Answer from the drawing. Dimensions are ordinates in mm from the lowest x, y and z of the part. A direction names the side the tool comes from. Coordinates: 2 decimals unless noted, no trailing zeros. Order: outer loops, then holes, each group sorted by start corner. A loop starts at its lowest first (then second) coordinate and runs counter-clockwise, first axis right, second up. Notation, with made-up numbers: (-23, 12) -> (14, 12) arc R30 ccw to (14, 39) -> close; hole circle Ø11 at (40.25, 52.25). An arc over 180 degrees is marked (long way). Answer in a Markdown table with one row per item.
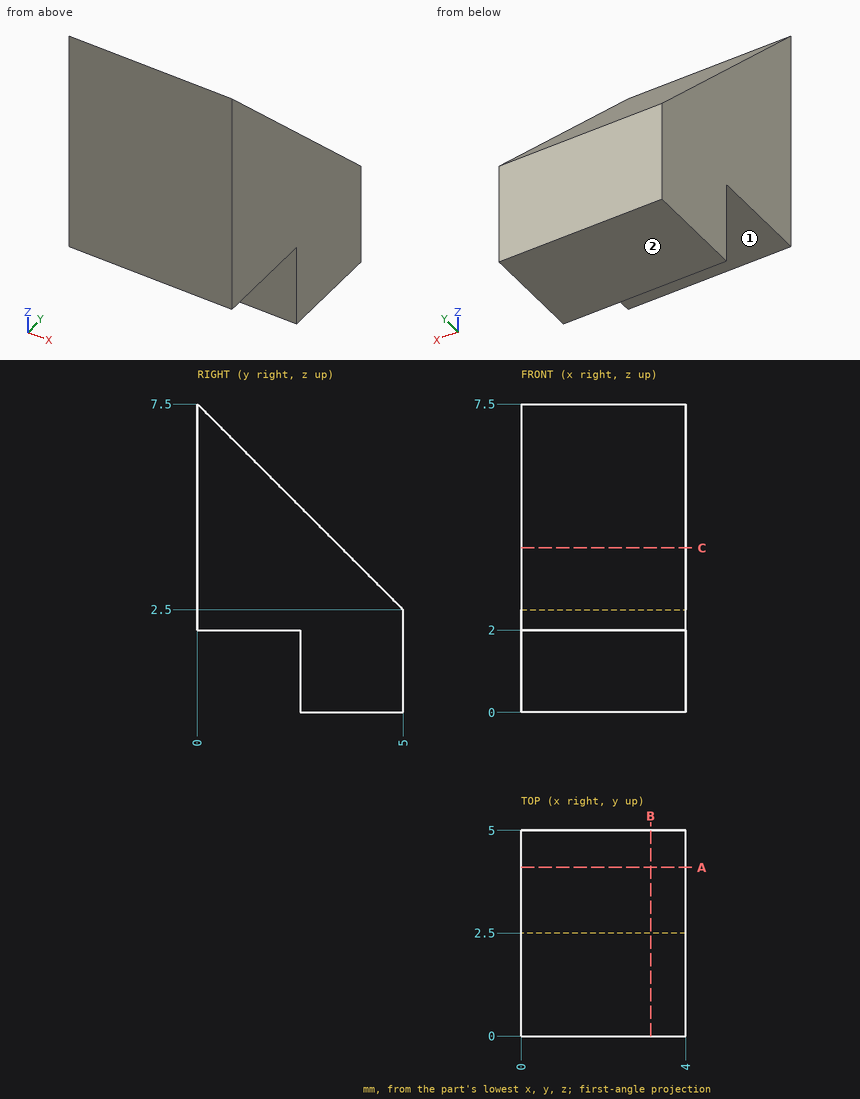
Q1. Consider line 1 (Y direction, x = 1.15, z = 0.5); line 2 (Y direction, x = 1.15, z = 5.5); line 3 (Z direction, x = 2.4, y = 4). Determine where each line is inside the solid, lowest interval first.
Outcome:
| item | result |
|---|---|
| line 1 | 2.5 to 5 |
| line 2 | 0 to 2 |
| line 3 | 0 to 3.5 |
Q2. Given pin 1 (1 mm diameter, centred on x = 1.5, z = 1, fed in from -Y); pin 2 (1.2 mm diameter, centred on x = 1.5, y = 1.5, fed in from -Z), each flat-ended and moving along its own axis, determine where each tip first touches the part or whether it passes through.
Outcome:
| item | result |
|---|---|
| pin 1 | y = 2.5 |
| pin 2 | z = 2 |
Q3. The part is cut by section A-A (y = 4.1). Write down the section's boundary in (x, z).
Outcome:
| item | result |
|---|---|
| outline | (0, 0) -> (4, 0) -> (4, 3.4) -> (0, 3.4) -> close |
Q4. The part is cut by section C-C (z = 4). Write down the section's boundary in (x, y), then the cut area to 3 significant figures.
Outcome:
| item | result |
|---|---|
| outline | (0, 0) -> (4, 0) -> (4, 3.5) -> (0, 3.5) -> close |
| area | 14.0 mm² |
Q5. For the marked faces 1 and 2, determine the directions among +Z, -Z, +X, -X, +Y, -Y from which every point of the face is accessible in a straight line to the end or side of a thin tool.
Outcome:
| item | result |
|---|---|
| face 1 | -Z, +X, -X, -Y |
| face 2 | -Z, +X, -X, +Y, -Y |
Q6. The part is cut by section B-B (x = 3.15). Write down the section's boundary in (y, z), then the cut area to 3 significant figures.
Outcome:
| item | result |
|---|---|
| outline | (0, 2) -> (2.5, 2) -> (2.5, 0) -> (5, 0) -> (5, 2.5) -> (0, 7.5) -> close |
| area | 20.0 mm² |
